Could you check a few things on this model? Use its own coordinates, in mm. Face numbers are marked on the shaded views. A direction names the side the tool comes from. Give positions to 0.01 mm unless a question says otherwise; leave off trailing zeros. Loops run counter-clockwise (first coordinate to the right, second up) from the corner with the lowest first, then second, coordinate; pieces in that order, holes last. Notation, with made-up numbers: M 56,1 L 74,1 A27 cw 74,35 Z; hole C -26,58.25 d4. An arc over 180 degrees is marked long. Answer in a Markdown table with one row per item. Add a question column.
```python
from build123d import *

# Parameters (mm, degrees)
CIRCLE_R         = 3.75
EXTRUDE001_DEPTH = 1.5
CIRCLE001_R      = 3.1
EXTRUDE_DEPTH    = 10
BOX_W            = 7.5
BOX_H            = 7.5
BOX_DEPTH        = 1


with BuildPart() as extrude001:
    # Circle → Extrude001 (new body)
    with BuildSketch(Plane(origin=(3.75, 3.75, 1), x_dir=(-1, 0, 0), z_dir=(0, 0, 1))):
        Circle(CIRCLE_R)
    extrude(amount=EXTRUDE001_DEPTH)


with BuildPart() as extrude001_1:
    # Extrude001 placement: moved
    add(extrude001.part.moved(Location((0, 0, -1.5))))


with BuildPart() as fusion:
    # Circle001 → Extrude (new body)
    with BuildSketch(Plane(origin=(3.75, 3.75, 1), x_dir=(-1, 0, 0), z_dir=(0, 0, 1))):
        Circle(CIRCLE001_R)
    extrude(amount=EXTRUDE_DEPTH)


with BuildPart() as fusion_1:
    # Extrude placement: moved
    add(fusion.part.moved(Location((0, 0, -10))))

    # Fusion: union Extrude001
    add(extrude001_1.part)


with BuildPart() as obj1:
    # Box → Box (new body)
    with BuildSketch(Plane.XY):
        with Locations((3.75, 3.75)):
            Rectangle(BOX_W, BOX_H)
    extrude(amount=BOX_DEPTH)

    # Fusion001: union Fusion
    add(fusion_1.part)


solid = obj1.part
```
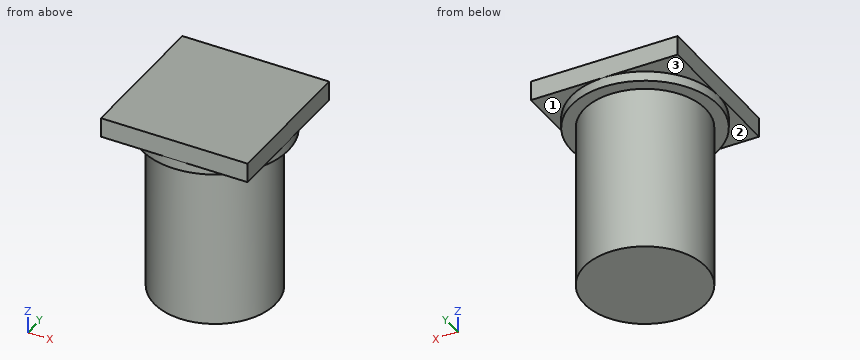
Item 1: I need wall thicknesses on L1, parallel to Z at x = 0.75, y = 2.5; L2, parallel to Y at x = 3.75, z = -2; L3, parallel to Z at x = 6.75, y = 1. Which ranges of each line are inside material? Lowest first, please.
Item 2: For P1, Ø2, axis at x = 1.5, z = -4.5, coming from the +Y side; P2, Ø1, axis at y = 2, z = -3.5, coming from the +X side, each with a flat end and sliding along its axis, tell me the tip position at first contact or that it passes through.
Item 3: Suppose I cut it at A-A (x = 1). List the corners of the cut face in (y, z) for me.
Item 4: Suppose I cut it at C-C (z = -5). List the corners of the cut face in (x, y) for me, then the cut area to 3 significant figures.
Item 5: Suppose I cut it at D-D (y = 0.5). List the corners of the cut face in (x, z) for me, then the cut area to 3 significant figures.
Item 6: For the marked faces 1, 2 and 3, which set-ups out of +Z, -Z, +X, -X, +Y, -Y let a thin tool reach every point of the face, with its end or its side?
Values found:
| question | item | result |
|---|---|---|
| 1 | L1 | -0.5 to 1 |
| 1 | L2 | 0.65 to 6.85 |
| 1 | L3 | 0 to 1 |
| 2 | P1 | y = 6.59 |
| 2 | P2 | x = 6.59 |
| 3 | outline | M 0,0 L 1.2,0 L 1.2,-0.5 L 2.32,-0.5 L 2.32,-9 L 5.18,-9 L 5.18,-0.5 L 6.3,-0.5 L 6.3,0 L 7.5,0 L 7.5,1 L 0,1 Z |
| 4 | outline | C 3.75,3.75 d6.2 |
| 4 | area | 30.2 mm² |
| 5 | outline | M 0,0 L 1.88,0 L 1.88,-0.5 L 5.62,-0.5 L 5.62,0 L 7.5,0 L 7.5,1 L 0,1 Z |
| 5 | area | 9.37 mm² |
| 6 | face 1 | -Z, +X, +Y |
| 6 | face 2 | -Z, -X, -Y |
| 6 | face 3 | -Z, -X, +Y |
